Source: CAD feature listing. Evaluate the final solid. Frame: model axes, mm. A direction names the side the tool comes from. Coordinates: 2 decimals unless noted, no trailing zeros. Loops run counter-clockwise (first coordinate to the right, second up) from the corner with the lowest first, then second, coordinate; pieces in that order, holes last.
```python
from build123d import *

# Parameters (mm, degrees)
SKETCH_1_W               = 160
SKETCH_1_H               = 185
EXTRUDE_1_DEPTH          = 10
EXTRUDE_2_DEPTH          = 80
SKETCH_14_W              = 20
SKETCH_14_H              = 50
CUT_EXTRUDE_4_DEPTH      = 258.342184649
SKETCH_16_W              = 32
SKETCH_16_H              = 20
EXTRUDE_7_DEPTH          = 5
CUT_EXTRUDE_7_REACH      = 262.624
SKETCH_18_R              = 3
FILLET_1_R               = 2
SKETCH_21_W              = 70
SKETCH_21_H              = 185
SKETCH_21_R              = 2.5
EXTRUDE_8_DEPTH          = 160
CUT_EXTRUDE_9_DEPTH      = 255.263642702
CUT_EXTRUDE_9_DEPTH_BACK = 255.263642702
SKETCH_23_W              = 122
SKETCH_23_H              = 70
CUT_EXTRUDE_10_DEPTH     = 258.342184649
CUT_EXTRUDE_11_REACH     = 259.342
SKETCH_24_W              = 5
SKETCH_24_H              = 20


with BuildPart() as part:
    # 草圖1 → 填料-伸長1 (new body)
    with BuildSketch(Plane.XY):
        with Locations((-80, -92.5)):
            Rectangle(SKETCH_1_W, SKETCH_1_H)
    extrude(amount=EXTRUDE_1_DEPTH)

    # 草圖2 → 填料-伸長2 (add)
    with BuildSketch(Plane(origin=(0, 0, 0), x_dir=(-1, 0, 0), z_dir=(0, 0, -1))):
        Polygon((0, 0), (0, -185), (5, -185), (5, -10), (155, -10), (155, -185), (160, -185), (160, 0), align=None)
    extrude(amount=EXTRUDE_2_DEPTH)

    # 草圖14 → 除料-伸長4 (cut, through all)
    with BuildSketch(Plane(origin=(0, 0, 0), x_dir=(1, 0, 0), z_dir=(0, 1, 0))):
        with Locations((-80, 5)):
            Rectangle(SKETCH_14_W, SKETCH_14_H)
    extrude(amount=-CUT_EXTRUDE_4_DEPTH, mode=Mode.SUBTRACT)

    # 草圖16 → 填料-伸長7 (add)
    with BuildSketch(Plane(origin=(0, 0, -80), x_dir=(-1, 0, 0), z_dir=(0, 0, -1))):
        with Locations((80, 10)):
            Rectangle(SKETCH_16_W, SKETCH_16_H)
    extrude(amount=-EXTRUDE_7_DEPTH)

    # 草圖18 → 除料-伸長7 (cut, up to next)
    with BuildSketch(Plane(origin=(0, 0, -80), x_dir=(-1, 0, 0), z_dir=(0, 0, -1)), mode=Mode.PRIVATE) as cut_extrude_7_sk1:
        with Locations((69, 12)):
            Circle(SKETCH_18_R)
    cut_extrude_7_tool1 = extrude(cut_extrude_7_sk1.sketch, amount=-CUT_EXTRUDE_7_REACH, mode=Mode.PRIVATE) & part.part
    # 草圖18 → 除料-伸長7 (cut, up to next)
    with BuildSketch(Plane(origin=(0, 0, -80), x_dir=(-1, 0, 0), z_dir=(0, 0, -1)), mode=Mode.PRIVATE) as cut_extrude_7_sk2:
        with Locations((91, 12)):
            Circle(SKETCH_18_R)
    cut_extrude_7_tool2 = extrude(cut_extrude_7_sk2.sketch, amount=-CUT_EXTRUDE_7_REACH, mode=Mode.PRIVATE) & part.part
    add(cut_extrude_7_tool1.solids().sort_by_distance((-69, 12, -80))[0], mode=Mode.SUBTRACT)
    add(cut_extrude_7_tool2.solids().sort_by_distance((-91, 12, -80))[0], mode=Mode.SUBTRACT)

    # 圓角1
    fillet_1_edges = [part.edges().sort_by_distance(p)[0] for p in [
        (-80, 0, -75),
        (-96, 0, -77.5),
        (-64, 0, -77.5),
    ]]
    fillet(fillet_1_edges, radius=FILLET_1_R)

    # 草圖21 → 填料-伸長8 (add)
    with BuildSketch(Plane.ZY.offset(160)):
        with Locations((45, -92.5)):
            Rectangle(SKETCH_21_W, SKETCH_21_H)
        with Locations((60, -10)):
            Circle(SKETCH_21_R, mode=Mode.SUBTRACT)
        with Locations((60, -175)):
            Circle(SKETCH_21_R, mode=Mode.SUBTRACT)
        with Locations((60, -34)):
            Circle(SKETCH_21_R, mode=Mode.SUBTRACT)
    extrude(amount=-EXTRUDE_8_DEPTH)

    # 草圖22 → 除料-伸長9 (cut, two sides: drawn at the far end of the back side and taken through both)
    with BuildSketch(Plane(origin=(-155, 0, 0), x_dir=(0, 0, -1), z_dir=(1, 0, 0)).offset(-CUT_EXTRUDE_9_DEPTH_BACK)):
        with BuildLine():
            Line((22.5, -98.5), (67.5, -98.5))
            ThreePointArc((67.5, -98.5), (69, -100), (67.5, -101.5))
            Line((67.5, -101.5), (22.5, -101.5))
            ThreePointArc((22.5, -101.5), (21, -100), (22.5, -98.5))
        make_face()
    extrude(amount=CUT_EXTRUDE_9_DEPTH + CUT_EXTRUDE_9_DEPTH_BACK, mode=Mode.SUBTRACT)

    # 草圖23 → 除料-伸長10 (cut, through all)
    with BuildSketch(Plane(origin=(0, 0, 0), x_dir=(1, 0, 0), z_dir=(0, 1, 0))):
        with Locations((-80, -45)):
            Rectangle(SKETCH_23_W, SKETCH_23_H)
    extrude(amount=-CUT_EXTRUDE_10_DEPTH, mode=Mode.SUBTRACT)

    # 草圖24 → 除料-伸長11 (cut, up to next)
    with BuildSketch(Plane(origin=(0, 0, 0), x_dir=(1, 0, 0), z_dir=(0, 1, 0)), mode=Mode.PRIVATE) as cut_extrude_11_sk1:
        with Locations((-142.5, 65)):
            Rectangle(SKETCH_24_W, SKETCH_24_H)
    cut_extrude_11_tool1 = extrude(cut_extrude_11_sk1.sketch, amount=-CUT_EXTRUDE_11_REACH, mode=Mode.PRIVATE) & part.part
    # 草圖24 → 除料-伸長11 (cut, up to next)
    with BuildSketch(Plane(origin=(0, 0, 0), x_dir=(1, 0, 0), z_dir=(0, 1, 0)), mode=Mode.PRIVATE) as cut_extrude_11_sk2:
        with Locations((-17.5, 65)):
            Rectangle(SKETCH_24_W, SKETCH_24_H)
    cut_extrude_11_tool2 = extrude(cut_extrude_11_sk2.sketch, amount=-CUT_EXTRUDE_11_REACH, mode=Mode.PRIVATE) & part.part
    add(cut_extrude_11_tool1.solids().sort_by_distance((-142.5, 0, -65))[0], mode=Mode.SUBTRACT)
    add(cut_extrude_11_tool2.solids().sort_by_distance((-17.5, 0, -65))[0], mode=Mode.SUBTRACT)


solid = part.part
```
Q1. Section query B-B on y = -127. Return the cut outline in (x, z).
Q2. Section query D-D on z = -6.5. Return the cut outline in (x, y).
Q3. Section query C-C on y = 12. Return the cut outline in (x, z).
Q4. Section query A-A on z = 60. Count the separate pieces of the cut face and the enclosed holes in it, then the cut area to 3 significant figures.
Q5. Reachability of faces 4 (the flat face through (-45, -91, 10)), 5 (the flat face through (-80, 11, -75)), 6 (the flat face through (-18, -5, -75)), 7 (the flat face through (-38, -96, 0)) from +Z, -Z, +X, -X, +Y, -Y: full face, straight path, thin tool, end or side. Return the list, or none.
Q6. First-contact query: pin 1 Ø2.5 at (x, z) = (-156.5, -46) entering from +Y; pin 2 Ø3 at (x, y) = (-124.5, -42.5) entering from -Z; pin 3 Ø1.5 at (x, z) = (-106, -18) entering from -Y; pin 4 Ø8 at (y, z) = (-7, -62.5) entering from +X. Flat tips, straight axial feed; report the tip coordinate or a pass-through.
Q7. Material intervals for line 1 along Y through (x, z) = (-154, 60); line 2 along X through (y, z) = (-13.5, 63); line 3 along X through (y, z) = (-108, -68), sorted ascending.
Q8. Draft query along X for faces 1 (the cylindrical face through (-9.63, -10.96, 62.31)), 2 (the flat face through (-18, -5, -55)), 3 (the flat face through (0, -91, -1)). Return one class per face: released by +X, released by -X, zero draft, split by the parting line, or undercut.
Resolved:
1. outline: (-160, -80) - (-155, -80) - (-155, 0) - (-90, 0) - (-90, 10) - (-141, 10) - (-141, 80) - (-160, 80) - close; (-70, 0) - (-5, 0) - (-5, -80) - (0, -80) - (0, 80) - (-19, 80) - (-19, 10) - (-70, 10) - close
2. outline: (-160, -185) - (-155, -185) - (-155, -10) - (-90, -10) - (-90, 0) - (-160, 0) - close; (-70, -10) - (-5, -10) - (-5, -185) - (0, -185) - (0, 0) - (-70, 0) - close
3. outline: (-96, -80) - (-94, -80) - (-94, -75) - (-96, -75) - close; (-88, -80) - (-72, -80) - (-72, -75) - (-88, -75) - close; (-66, -80) - (-64, -80) - (-64, -75) - (-66, -75) - close
4. separate pieces: 8
4. enclosed holes: 0
4. area: 6,460 mm2
5. face 4: +Z, +Y, -Y
5. face 5: +Z, +X, -X, +Y
5. face 6: +Y, -Y
5. face 7: -Z, -Y
6. pin 1: stops at y = 0
6. pin 2: stops at z = 0
6. pin 3: stops at y = -10
6. pin 4: stops at x = 0
7. line 1: y = -185 to -177.5, -172.5 to -36.5, -31.5 to -12.5, -7.5 to 0
7. line 2: x = -160 to -141, -19 to 0
7. line 3: x = -160 to -155, -5 to 0
8. face 1: zero draft
8. face 2: undercut
8. face 3: released by +X
